from build123d import *

# Parameters (mm, degrees)
F0_R     = 25
F1_DEPTH = 25
F2_R     = 24.99999
F3_R     = 26.5
F3_R_2   = 24.5
F4_DEPTH = 25


# Not quite as in the source:
# - a fillet or chamfer is up to 0.001 mm smaller than in the source, because OpenCascade refuses the exact size


with BuildPart() as f1:
    # F0 (on Top) → F1 (new body)
    with BuildSketch(Plane.XY):
        with Locations((-7.374277804, 10.7427751645)):
            Circle(F0_R)
    extrude(amount=F1_DEPTH)

    # F2 (radius 25 in the source; OpenCascade refuses exactly that, so slightly less here)
    f2_edges = [f1.edges().sort_by_distance(p)[0] for p in [
        (-32.374278, 10.742775, 25),
    ]]
    fillet(f2_edges, radius=F2_R)

    # F3 (on Top) → F4 (join)
    with BuildSketch(Plane.XY):
        with Locations((-7.374277804, 10.7427751645)):
            Circle(F3_R)
        with Locations((-7.374277804, 10.7427751645)):
            Circle(F3_R_2, mode=Mode.SUBTRACT)
    extrude(amount=F4_DEPTH)


solid = f1.part
Read the model definition and answer for the solid it produces. Units are mm, in the model's axes. Give positions to 0.01 mm unless a question says otherwise; leave off trailing zeros. Write each question's results on one line, items separated by ' | '.
1. Given pin 1 (6 mm diameter, centred on y = -9, z = 16, fed in from +X); pin 2 (10 mm diameter, centred on x = -23, y = 8, fed in from +Z); pin 3 (1 mm diameter, centred on x = 4, y = 21, fed in from +Z), each flat-ended and moving along its own axis, determine where each tip first touches the part or whether it passes through.
Values:
pin 1: stops at x = 13.17 | pin 2: stops at z = 22.52 | pin 3: stops at z = 20.14
2. Section A-A on z = 7 is taken. State how many separate pieces and enclosed holes the cut face has, plus the area to 3 significant figures.
Values:
separate pieces: 2 | enclosed holes: 1 | area: 2,130 mm^2
3. A straight line is drawn through the part: line 1 (Y direction, x = 9.5, z = 16). Find the intervals that lie inside material, in ascending order. Write a range as [from, to].
Values:
line 1: y = [-9.69, -7.02], [1.56, 19.92], [28.51, 31.18]
